The model under review builds one solid part; all positions refer to its coordinate system, in mm. A direction names the side the tool comes from. Coordinates: 2 decimals unless noted, no trailing zeros. Order: outer loops, then holes, each group sorted by start corner. A loop starts at its lowest first (then second) coordinate and runs counter-clockwise, first axis right, second up. Notation, with made-up numbers: (54.5, 13) -> (97.5, 13) arc R18 cw to (97.5, 38) -> close; hole circle Ø5 at (86, 38). An arc over 180 degrees is marked (long way). Use one line per item in the form item = value.
from build123d import *

# Parameters (mm, degrees)
SKETCH_1_R      = 1.45
EXTRUDE_1_DEPTH = 3.3
SKETCH_2_R      = 1.9
EXTRUDE_2_DEPTH = 1
SKETCH_3_R      = 0.25
EXTRUDE_3_DEPTH = 12.7


with BuildPart() as part:
    # 草图1 → 拉伸1 (new body)
    with BuildSketch(Plane.XY):
        Circle(SKETCH_1_R)
    extrude(amount=EXTRUDE_1_DEPTH)

    # 草图2 → 拉伸2 (add)
    with BuildSketch(Plane.XY.offset(3.3)):
        Circle(SKETCH_2_R)
    extrude(amount=EXTRUDE_2_DEPTH)

    # 草图3 → 拉伸3 (add)
    with BuildSketch(Plane.XY.offset(4.3)):
        with Locations((-1.27, 0)):
            Circle(SKETCH_3_R)
        with Locations(Location((1.27, 0, 0), (0, 0, 180))):
            Circle(SKETCH_3_R)
    extrude(amount=EXTRUDE_3_DEPTH)


solid = part.part
Item 1: Tool access review of faces 1 (the face through (-1.45, 0.06, 1.63)), 2 (the face through (-1.9, 0.08, 3.79)): name each direction out of +Z, -Z, +X, -X, +Y, -Y from which nothing blocks a thin tool from reaching the whole face with its end or side.
Results found:
face_1 = -Z
face_2 = +Z, -Z
Item 2: We need section C-C (y = 0). Write out the cut boundary in (x, z).
Results found:
outline = (-1.9, 3.3) -> (-1.45, 3.3) -> (-1.45, 0) -> (1.45, 0) -> (1.45, 3.3) -> (1.9, 3.3) -> (1.9, 4.3) -> (1.52, 4.3) -> (1.52, 17) -> (1.02, 17) -> (1.02, 4.3) -> (-1.02, 4.3) -> (-1.02, 17) -> (-1.52, 17) -> (-1.52, 4.3) -> (-1.9, 4.3) -> close
Item 3: We need section B-B (x = 0). Write out the cut boundary in (y, z).
Results found:
outline = (-1.9, 3.3) -> (-1.45, 3.3) -> (-1.45, 0) -> (1.45, 0) -> (1.45, 3.3) -> (1.9, 3.3) -> (1.9, 4.3) -> (-1.9, 4.3) -> close
Item 4: We need section D-D (x = 1.27). Write out the cut boundary in (y, z).
Results found:
outline = (-1.41, 3.3) -> (-0.7, 3.3) -> (-0.7, 0) -> (0.7, 0) -> (0.7, 3.3) -> (1.41, 3.3) -> (1.41, 4.3) -> (0.25, 4.3) -> (0.25, 17) -> (-0.25, 17) -> (-0.25, 4.3) -> (-1.41, 4.3) -> close
Item 5: To check wall thickness, follow L1, parallel to Z at x = 0.7, y = -0.9; L2, parallel to Z at x = 0, y = -1.5; L3, parallel to X at y = 0.1, z = 9.25. State the ranges of each line that lie inside material, in increasing order. Write a range as from..to.
Results found:
L1 = 0..4.3
L2 = 3.3..4.3
L3 = -1.5..-1.04, 1.04..1.5
Item 6: Clearance check with a flat-ended pin moving along its axis: pin 1 (2 mm diameter, centred on y = -0.5, z = 8, fed in from +X). State where the tip first meets the part, or that it passes through.
Results found:
pin_1 = 1.52
Item 7: We need section A-A (z = 16). Write out the cut boundary in (x, y).
Results found:
outline = circle Ø0.5 at (-1.27, 0); circle Ø0.5 at (1.27, 0)
